```python
from build123d import *

# Parameters (mm, degrees)
F0_W      = 20
F0_H      = 70
F1_DEPTH  = 30
F2_W      = 30
F2_H      = 10
F3_DEPTH  = 10
F4_R      = 2.05
F5_DEPTH  = 10
F6_W      = 11
F6_H      = 30
F7_DEPTH  = 50
F9_DEPTH  = 5
F10_SIZE2 = 10.99999
F10_SIZE  = 49.99999
F11_W     = 30
F11_H     = 10
F12_DEPTH = 25


# Not quite as in the source:
# - a fillet or chamfer is up to 0.001 mm smaller than in the source, because OpenCascade refuses the exact size


with BuildPart() as f1:
    # F0 (on Front) → F1 (new body)
    with BuildSketch(Plane.XZ):
        with Locations((-10, 35)):
            Rectangle(F0_W, F0_H)
    extrude(amount=F1_DEPTH)

    # F2 (on face) → F3 (cut)
    with BuildSketch(Plane(origin=(-20, 0, 0), x_dir=(0, -1, 0), z_dir=(-1, 0, 0))):
        with Locations((15, 5)):
            Rectangle(F2_W, F2_H)
    extrude(amount=-F3_DEPTH, mode=Mode.SUBTRACT)

    # F4 (on face) → F5 (cut, through all)
    with BuildSketch(Plane(origin=(-10, 0, 0), x_dir=(0, -1, 0), z_dir=(-1, 0, 0))):
        with Locations((5, 5)):
            Circle(F4_R)
        with Locations((25, 5)):
            Circle(F4_R)
    extrude(amount=-F5_DEPTH, mode=Mode.SUBTRACT)

    # F6 (on face) → F7 (cut)
    with BuildSketch(Plane.XY.offset(70)):
        with Locations((-5.5, -15)):
            Rectangle(F6_W, F6_H)
    extrude(amount=-F7_DEPTH, mode=Mode.SUBTRACT)

    # F8 (on face) → F9 (join)
    with BuildSketch(Plane.XY.offset(70)):
        with BuildLine():
            ThreePointArc((-17, -11.0388736054), (-19.25, -7), (-17, -2.9611263946))
            Line((-17, -2.9611263946), (-17, 0))
            Line((-17, 0), (-20, 0))
            Line((-20, 0), (-20, -30))
            Line((-20, -30), (-17, -30))
            Line((-17, -30), (-17, -27.0388736054))
            ThreePointArc((-17, -27.0388736054), (-19.25, -23), (-17, -18.9611263946))
            Line((-17, -18.9611263946), (-17, -11.0388736054))
        make_face()
    extrude(amount=F9_DEPTH)

    # F10 (size 50 and 11 in the source; OpenCascade refuses exactly that, so slightly less here)
    f10_edges = [f1.edges().sort_by_distance(p)[0] for p in [
        (-11, -15, 20),
    ]]
    f10_side = f1.faces().sort_by_distance((-11, -15, 45))[0]
    chamfer(f10_edges, length=F10_SIZE, length2=F10_SIZE2, reference=f10_side)

    # F11 (on face) → F12 (cut)
    with BuildSketch(Plane(origin=(-10, 0, 0), x_dir=(0, -1, 0), z_dir=(-1, 0, 0))):
        with Locations((15, 5)):
            Rectangle(F11_W, F11_H)
    extrude(amount=-F12_DEPTH, mode=Mode.SUBTRACT)


solid = f1.part
```
Build history of the part. All positions in model axes, mm. A direction names the side the tool comes from. Coordinates: 2 decimals unless noted, no trailing zeros. Order: outer loops, then holes, each group sorted by start corner. A loop starts at its lowest first (then second) coordinate and runs counter-clockwise, first axis right, second up. Notation, with made-up numbers: (3, -14.75) -> (19, -14.75) arc R26 cw to (19, 4.25) -> close; hole circle Ø9 at (1.5, -23.75). An arc over 180 degrees is marked (long way). Answer in a Markdown table with one row per item. Add a question column.
Q1. Which spindle directions (+Z, -Z, +X, -X, +Y, -Y) get a long thin tool onto all of the face, cutting with end or side? Do faces 4 (the face through (-19.25, -7.07, 72.46)), 5 (the face through (-17, -29, 72)), 6 (the face through (-12, 0, 35)). Say none if no direction does.
Q2. Drop flat-ended pins along their axis: pin 1 (5.5 mm diameter, centred on y = -13.5, z = 73, fed in from +X); pin 2 (6 mm diameter, centred on x = -11, y = -5.5, fed in from +Z); pin 3 (12 mm diameter, centred on y = -20.5, z = 49, fed in from +X); pin 4 (8 mm diameter, centred on x = -7, z = 56.5, fed in from +Y). Give the stop position or say it passes through.
Q3. Band-saw the part on C-C, the plane x = -12. List the corners of the cut face in (y, z), then the cut area to 3 significant figures.
Q4. Wall check: line 1 along Z through (x, y) = (-16.5, -25); line 2 along X through (y, z) = (-20.25, 51); line 3 along X through (y, z) = (-10.75, 22). Give the ranges that are in metal, low to high. Write a range as [from, to].
Q5. Band-saw the part on B-B, the plane z = 58. List the corners of the cut face in (x, y), then the cut area to 3 significant figures.
Q6. Mould opens along Y. For faces 1 (the face through (-12, -30, 36)), 2 (the face through (-14, -15, 70)), 3 (the face through (-5.423, -15.21, 44.65)) say: +Y half, -Y half, draft (parallel to the pull), parting line (faces both ways), or undercut.
Answers follow:
| question | item | result |
|---|---|---|
| 1 | face 4 | +Z, +X |
| 1 | face 5 | +Z, +X, +Y, -Y |
| 1 | face 6 | +Z, -Z, +X, -X, +Y |
| 2 | pin 1 | x = -17 |
| 2 | pin 2 | z = 70 |
| 2 | pin 3 | x = -5.06 |
| 2 | pin 4 | y = 0 |
| 3 | outline | (-30, 10) -> (0, 10) -> (0, 70) -> (-30, 70) -> close |
| 3 | area | 1,800 mm^2 |
| 4 | line 1 | [10, 70] |
| 4 | line 2 | [-20, -6.82] |
| 4 | line 3 | [-20, -0.44] |
| 5 | outline | (-20, -30) -> (-8.36, -30) -> (-8.36, 0) -> (-20, 0) -> close |
| 5 | area | 349 mm^2 |
| 6 | face 1 | -Y half |
| 6 | face 2 | undercut |
| 6 | face 3 | draft |
